Here's the drawing with two shaded views (mm, measured from the low corner). I have some questions. A direction names the side the tool comes from. Coordinates: 2 decimals unless noted, no trailing zeros. Loops run counter-clockwise (first coordinate to the right, second up) from the corner with the lowest first, then second, coordinate; pieces in that order, holes last. Notation, with made-up numbers: (84.25, 58) -> (96.25, 58) arc R28 ccw to (96.25, 87) -> close; hole circle Ø3 at (3, -1.5). An arc over 180 degrees is marked (long way). Answer as a JSON object with one key per item and string values. Group by question number.
1) I want a section at C-C (z = 518.5). Write out the boundary of the cut face in (x, y).
2) I want a section at B-B (y = 132). Write out the boundary of the cut face in (x, z), then the cut area to 3 significant figures.
3) I need wall thicknesses on probe 1 along X at (y, z) = (146.5, 437.5); probe 2 along Y at (x, z) = (677, 579.5); probe 3 along Z at (x, y) = (381.5, 294). Which ranges of each line are inside material? Lowest first, please. Write a range as [from, to].
4) I want a section at A-A (x = 113). Write out the boundary of the cut face in (y, z).
5) I want a section at D-D (x = 1321). Write out the boundary of the cut face in (y, z), then the cut area to 3 significant figures.
6) If we mould it in two halves opening along X, with no side actions, what happens to the marked faces 1, 2 and 3? For each: +X half, -X half, draft (parallel to the pull), parting line (faces both ways), or undercut.
7) Which directions (+Z, -Z, +X, -X, +Y, -Y) give clear straight access to the entire face, cutting with the end or side of a thin tool? Please do the marked faces 4, 5 and 6.
8) I'm going to push flat-ended pins straight in: pin 1 (2 mm diameter, centred on x = 911, z = 426, fed in from -Y); pin 2 (6 mm diameter, centred on y = 494.5, z = 435, fed in from -X); pin 3 (1.5 mm diameter, centred on x = 1233.5, y = 505.5, fed in from +Z). Where does each tip first touch, or does it pass through?
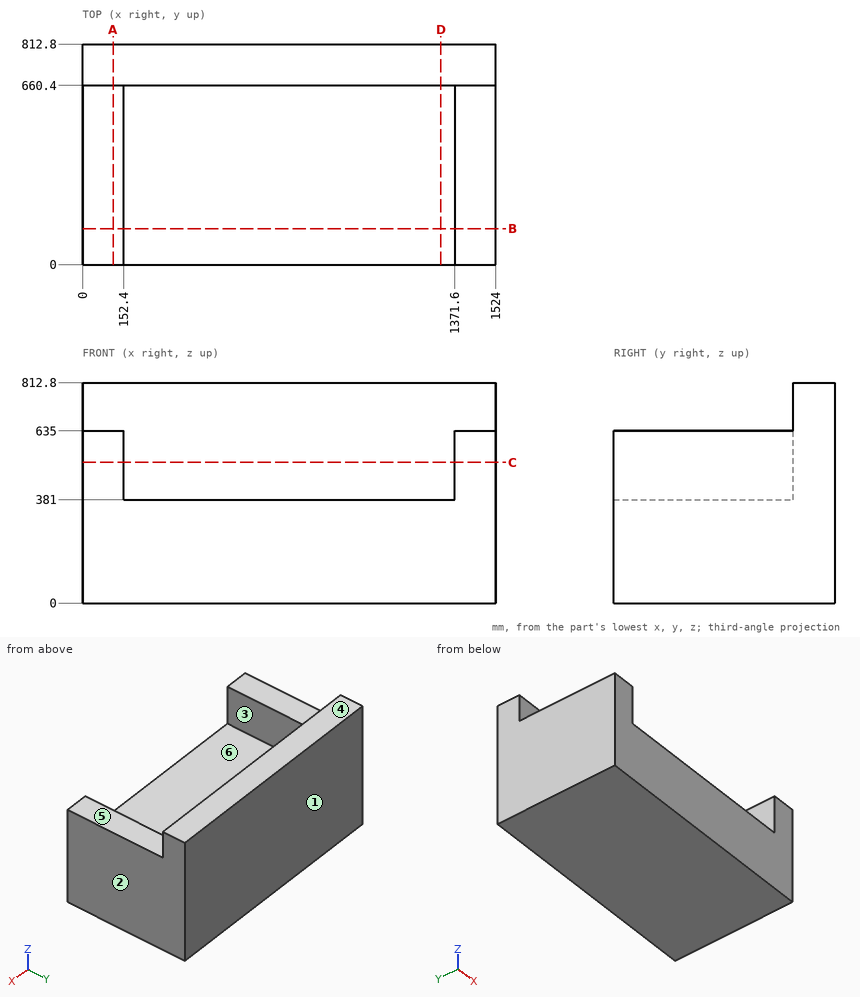
Determined:
{
 "1": {"outline": "(0, 0) -> (152.4, 0) -> (152.4, 660.4) -> (1371.6, 660.4) -> (1371.6, 0) -> (1524, 0) -> (1524, 812.8) -> (0, 812.8) -> close"},
 "2": {"outline": "(0, 0) -> (1524, 0) -> (1524, 635) -> (1371.6, 635) -> (1371.6, 381) -> (152.4, 381) -> (152.4, 635) -> (0, 635) -> close", "area": "658,000 mm^2"},
 "3": {"probe 1": "[0, 152.4], [1371.6, 1524]", "probe 2": "[660.4, 812.8]", "probe 3": "[0, 381]"},
 "4": {"outline": "(0, 0) -> (812.8, 0) -> (812.8, 812.8) -> (660.4, 812.8) -> (660.4, 635) -> (0, 635) -> close"},
 "5": {"outline": "(0, 0) -> (812.8, 0) -> (812.8, 812.8) -> (660.4, 812.8) -> (660.4, 381) -> (0, 381) -> close", "area": "375,000 mm^2"},
 "6": {"face 1": "draft", "face 2": "+X half", "face 3": "undercut"},
 "7": {"face 4": "+Z, +X, -X, +Y, -Y", "face 5": "+Z, +X, -X, -Y", "face 6": "+Z, -Y"},
 "8": {"pin 1": "y = 660.4", "pin 2": "x = 0", "pin 3": "z = 381"}
}
